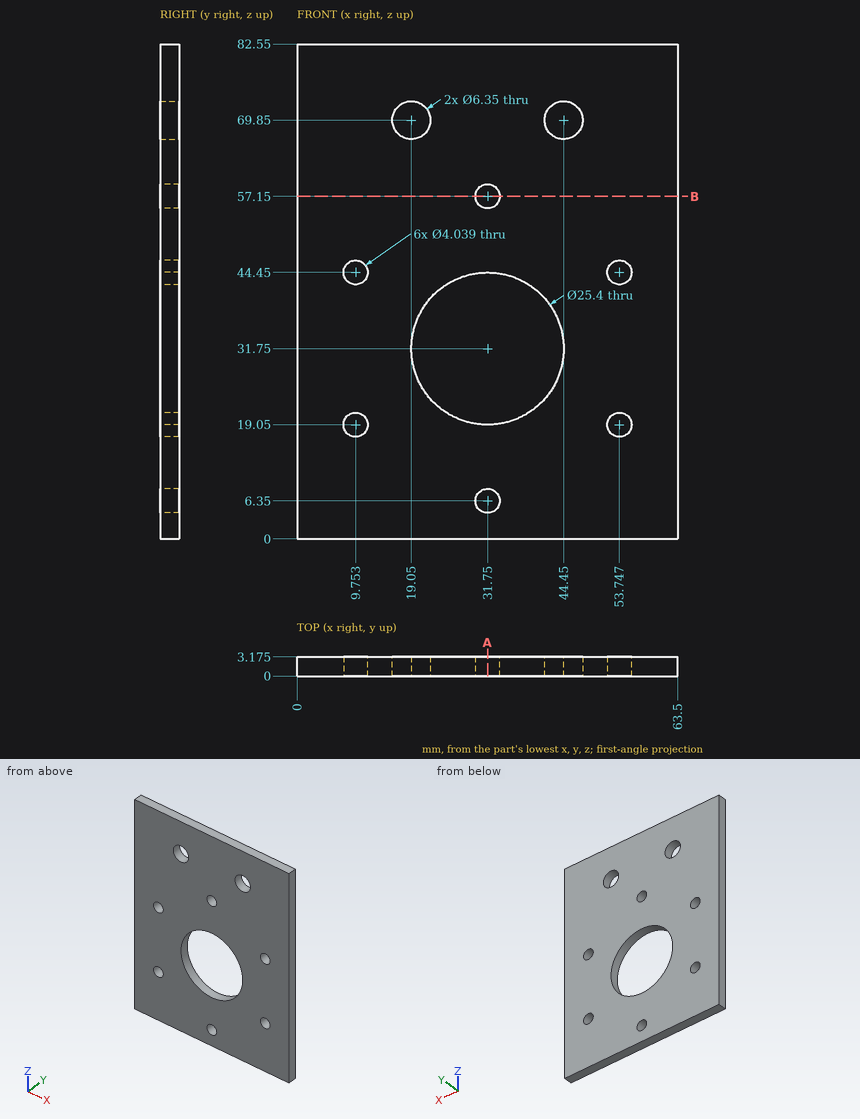
Check sheet for the drawn part. Datum: minimum x, y, z corner. Units: mm. Coordinates: 2 decimals unless noted, no trailing zeros. Write each loop counter-clockwise with the first axis right and the second up, starting at its lowest first coordinate (ties: lowest second). Pieces come first, ordered by that corner, then holes. Notation, with made-up numbers: M 30.25,11.25 L 41.25,11.25 A17 cw 41.25,43.25 Z; hole C 20,21.25 d3. An arc over 180 degrees is marked long. One line per item, written item: value.
Item 1: Section check A-A, the plane x = 31.75. State how many separate pieces and enclosed holes the cut face has, plus the area to 3 significant figures.
Check sheet entries:
separate pieces: 4
enclosed holes: 0
area: 156 mm^2
Item 2: Scan lines: line 1 along Z through (x, y) = (31.75, 2.5); line 2 along X through (y, z) = (1.95, 6.35); line 3 along X through (y, z) = (1.8, 69.85) (1 decimal). Record each from-to range of solid material in increasing order.
Check sheet entries:
line 1: z = 0 to 4.33, 8.37 to 19.05, 44.45 to 55.13, 59.17 to 82.55
line 2: x = 0 to 29.73, 33.77 to 63.5
line 3: x = 0 to 15.9, 22.2 to 41.3, 47.6 to 63.5
Item 3: Section check B-B, the plane z = 57.15. Record the boundary of the cut face in (x, y) (1 decimal), plus the area to 3 significant figures.
Check sheet entries:
outline: M 0,0 L 29.7,0 L 29.7,3.2 L 0,3.2 Z; M 33.8,0 L 63.5,0 L 63.5,3.2 L 33.8,3.2 Z
area: 189 mm^2
